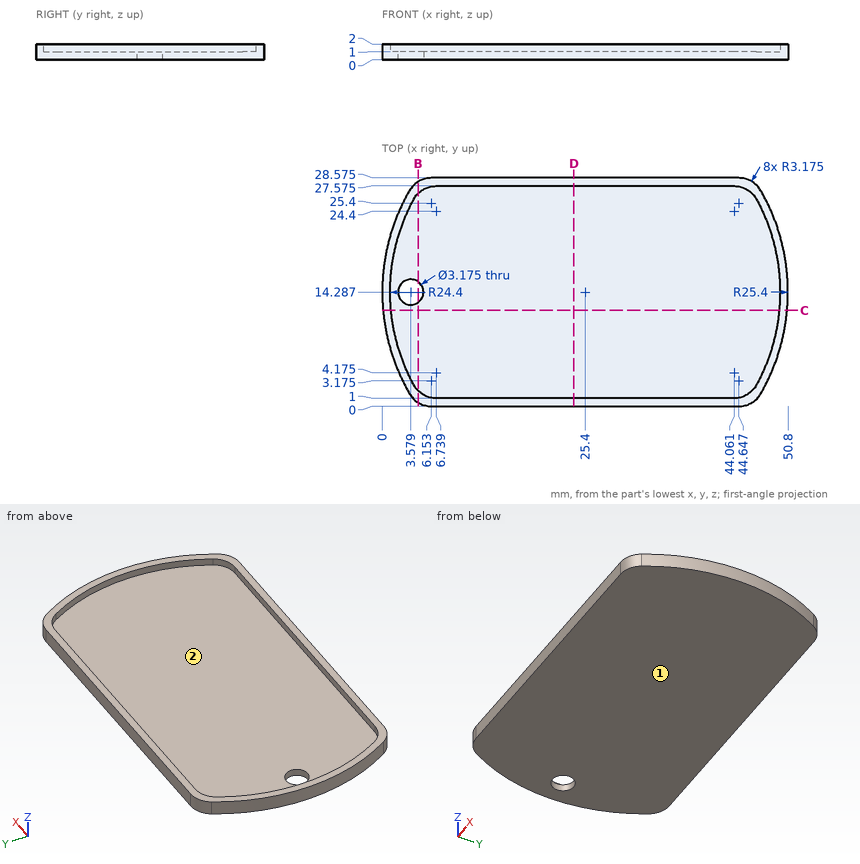
Job drawing, mm, ordinate dimensions from the low corner. One solid piece. Coordinates: 2 decimals unless noted, no trailing zeros. Write each loop counter-clockwise with the first axis right and the second up, starting at its lowest first coordinate (ties: lowest second). Pieces come first, ordered by that corner, then holes. Notation, with made-up numbers: (13, 22) - (71, 22) arc R11 ccw to (71, 42) - close; hole circle Ø11 at (-21.5, 33.25). An arc over 180 degrees is marked (long way). Use a Markdown table: item, result. Add a question column.
Item 1: Flat gauge pins, fed straight in: pin 1 (5 mm diameter, centred on x = 28.5, y = 16.5, fed in from +Z); pin 2 (2.5 mm diameter, centred on x = 3.58, y = 14.29, fed in from -Z). Where does each tip first touch, or does it go through?
Item 2: Band-saw the part on B-B, the plane x = 4.5. Give the cut face in (y, z) (1 decimal).
Item 3: Band-saw the part on D-D, the plane x = 24. Give the cut face in (y, z) (1 decimal).
Item 4: Drill centre lines: L1, parallel to Y at x = 25, z = 1.3 (1 decimal); L2, parallel to Z at x = 18, y = 8.75; L3, parallel to X at y = 18.5, z = 1.05. Where is each one in solid material? Low to high. Write a range as from..to.
Item 5: Band-saw the part on C-C, the plane y = 12. Give the cut face in (x, z).
Item 6: Mould opens along X. For the marked faces 1 and 2 say: pulls with the +X half, pulls with the -X half, needs draft (parallel to the pull), parting line crosses it, or undercut.
Numbers:
| question | item | result |
|---|---|---|
| 1 | pin 1 | z = 1 |
| 1 | pin 2 | through |
| 2 | outline | (0.5, 0) - (13, 0) - (13, 1) - (1.9, 1) - (1.9, 2) - (0.5, 2) - close; (15.6, 0) - (28.1, 0) - (28.1, 2) - (26.7, 2) - (26.7, 1) - (15.6, 1) - close |
| 3 | outline | (0, 0) - (28.6, 0) - (28.6, 2) - (27.6, 2) - (27.6, 1) - (1, 1) - (1, 2) - (0, 2) - close |
| 4 | L1 | 0..1, 27.6..28.6 |
| 4 | L2 | 0..1 |
| 4 | L3 | 0.35..1.37, 49.43..50.45 |
| 5 | outline | (0.1, 0) - (50.7, 0) - (50.7, 2) - (49.69, 2) - (49.69, 1) - (1.11, 1) - (1.11, 2) - (0.1, 2) - close |
| 6 | face 1 | needs draft |
| 6 | face 2 | undercut |
